```python
from build123d import *

# Parameters (mm, degrees)
SKETCH_1_R                   = 8.3
EXTRUDE_1_DEPTH              = 2.25
EXTRUDE_START                = 2
EXTRUDE_2_DEPTH              = 2
EXTRUDE_START_2              = 4.5
EXTRUDE_3_DEPTH              = 4.5
EXTRUDE_4_DEPTH              = 2
FILLET_1_R                   = 0.5
SKETCH_5_R                   = 1.85
EXTRUDE_5_DEPTH              = 0.5
HOLE_WIZARD_M2_1_D           = 2.1
HOLE_WIZARD_M2_1_CBORE_D     = 3.8
HOLE_WIZARD_M2_1_CBORE_DEPTH = 1
FILLET_2_R                   = 2


with BuildPart() as part:
    # ｽｹｯﾁ1 → ﾎﾞｽ - 押し出し1 (new body)
    with BuildSketch(Plane(origin=(0, 0, 0), x_dir=(1, 0, 0), z_dir=(0, 1, 0))):
        with BuildLine():
            ThreePointArc((13, 10.5), (0, 23.5), (-13, 10.5))
            Line((-13, 10.5), (-13, -13))
            Line((-13, -13), (13, -13))
            Line((13, -13), (13, 10.5))
        make_face()
        with Locations(Location((0, 10.5, 0), (0, 0, 270))):
            Circle(SKETCH_1_R, mode=Mode.SUBTRACT)
    extrude(amount=EXTRUDE_1_DEPTH)

    # ｽｹｯﾁ2 → ﾎﾞｽ - 押し出し2 (add)
    with BuildSketch(Plane.XZ.offset(EXTRUDE_START)):
        with BuildLine():
            Line((-12.649110641, -13.5), (-5.48292805, -13.5))
            ThreePointArc((-5.48292805, -13.5), (0, -16.75), (5.48292805, -13.5))
            Line((5.48292805, -13.5), (12.649110641, -13.5))
            ThreePointArc((12.649110641, -13.5), (0, -23.5), (-12.649110641, -13.5))
        make_face()
    extrude(amount=-EXTRUDE_2_DEPTH)

    # ｽｹｯﾁ3 → ﾎﾞｽ - 押し出し3 (add)
    with BuildSketch(Plane.XZ.offset(2).offset(EXTRUDE_START_2)):
        with BuildLine():
            Line((-9.38083152, -19.5), (-7.158910532, -19.5))
            ThreePointArc((-7.158910532, -19.5), (0, -22), (7.158910532, -19.5))
            Line((7.158910532, -19.5), (9.38083152, -19.5))
            ThreePointArc((9.38083152, -19.5), (0, -23.5), (-9.38083152, -19.5))
        make_face()
    extrude(amount=-EXTRUDE_3_DEPTH)

    # ｽｹｯﾁ4 → ﾎﾞｽ - 押し出し4 (add)
    with BuildSketch(Plane.XZ.offset(EXTRUDE_START)):
        with BuildLine():
            Line((-6.25, 6.25), (6.25, 6.25))
            Line((6.25, 6.25), (6.25, -10.5))
            ThreePointArc((6.25, -10.5), (0, -4.25), (-6.25, -10.5))
            Line((-6.25, -10.5), (-6.25, 6.25))
        make_face()
    extrude(amount=-EXTRUDE_4_DEPTH)

    # ﾌｨﾚｯﾄ1
    # the kernel refuses this fillet: 0.5 mm, written as the material it takes off along each edge
    with BuildSketch(Plane(origin=(5.48292805, -2.721925351, -13.5), x_dir=(1, 0, 0), z_dir=(0, 1, 0))) as fillet_1_piece_1:
        with BuildLine():
            CenterArc((0.28877014, 0.5), FILLET_1_R, 211.232929016, 58.767070984)
            ThreePointArc((-0.138763059, 0.240740741), (-0.068043475, 0.121141625), (0, 0))
            Line((0, 0), (0.28877014, 0))
        make_face()
    extrude(amount=3.443850702, mode=Mode.SUBTRACT)
    with BuildSketch(Plane(origin=(-5.48292805, -2.721925351, -13.5), x_dir=(-1, 0, 0), z_dir=(0, 1, 0))) as fillet_1_piece_2:
        with BuildLine():
            CenterArc((0.28877014, -0.5), FILLET_1_R, 90, 58.767070984)
            ThreePointArc((-0.138763059, -0.240740741), (-0.068043475, -0.121141625), (0, 0))
            Line((0, 0), (0.28877014, 0))
        make_face()
    extrude(amount=3.443850702, mode=Mode.SUBTRACT)
    with BuildSketch(Plane(origin=(-6.25, -10.838834765, -10.5), x_dir=(0, 0, 1), z_dir=(0, 1, 0))) as fillet_1_piece_3:
        with BuildLine():
            CenterArc((3.535533906, 0.5), FILLET_1_R, 121.586338097, 148.413661903)
            ThreePointArc((3.273642506, 0.925925926), (1.701034544, 0.235934696), (0, 0))
            Line((0, 0), (3.535533906, 0))
        make_face()
    extrude(amount=19.67766953, mode=Mode.SUBTRACT)
    with BuildSketch(Plane(origin=(6.25, -10.838834765, -10.5), x_dir=(0, 0, 1), z_dir=(0, 1, 0))) as fillet_1_piece_4:
        with BuildLine():
            CenterArc((3.535533906, -0.5), FILLET_1_R, 90, 148.413661903)
            ThreePointArc((3.273642506, -0.925925926), (1.701034544, -0.235934696), (0, 0))
            Line((0, 0), (3.535533906, 0))
        make_face()
    extrude(amount=19.67766953, mode=Mode.SUBTRACT)

    # ｽｹｯﾁ5 → ﾎﾞｽ - 押し出し5 (add)
    with BuildSketch(Plane.XZ):
        with Locations(Location((-10.5, 10.5, 0), (0, 0, 90))):
            Circle(SKETCH_5_R)
        with Locations(Location((10.5, 10.5, 0), (0, 0, 90))):
            Circle(SKETCH_5_R)
        with Locations(Location((-10.5, -10.5, 0), (0, 0, 90))):
            Circle(SKETCH_5_R)
        with Locations(Location((10.5, -10.5, 0), (0, 0, 90))):
            Circle(SKETCH_5_R)
    extrude(amount=EXTRUDE_5_DEPTH)

    # M2 丸平ねじ用座ぐり穴1 (through all)
    with Locations(Plane(origin=(0, 2.25, 0), x_dir=(1, 0, 0), z_dir=(0, 1, 0))):
        with Locations((10.5, 10.5), (-10.5, 10.5), (-10.5, -10.5), (10.5, -10.5)):
            CounterBoreHole(HOLE_WIZARD_M2_1_D / 2, HOLE_WIZARD_M2_1_CBORE_D / 2, HOLE_WIZARD_M2_1_CBORE_DEPTH)

    # ﾌｨﾚｯﾄ2
    fillet_2_edges = [part.edges().sort_by_distance(p)[0] for p in [
        (13, 1.125, 13),
        (-13, 1.125, 13),
    ]]
    fillet(fillet_2_edges, radius=FILLET_2_R)


solid = part.part
```
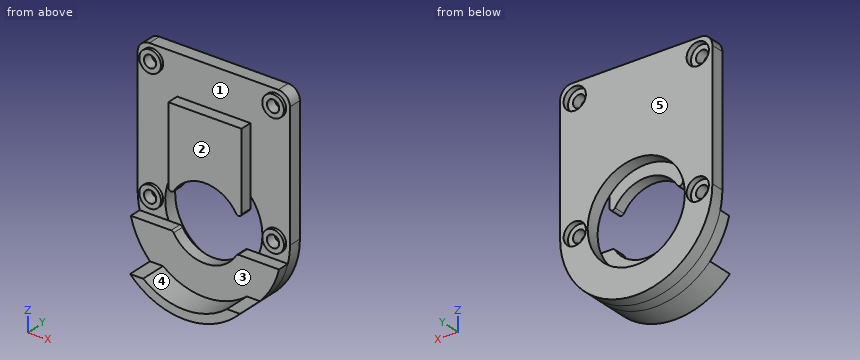
Source: CAD feature listing. Evaluate the final solid. Frame: model axes, mm. Face numbers are marked on the shaded views. A direction names the side the tool comes from. Coordinates: 2 decimals unless noted, no trailing zeros. Write each loop counter-clockwise with the first axis right and the second up, starting at its lowest first coordinate (ties: lowest second). Pieces come first, ordered by that corner, then holes. Notation, with made-up numbers: M 16.25,9.25 L 45.25,9.25 A26 ccw 45.25,36.25 Z; hole C -8.5,25.25 d6. An arc over 180 degrees is marked long. Answer as a JSON object with one key per item and string values.
1. Contact query for flat-ended pins moving along their axis: P1, Ø6, axis at x = 10.5, z = -10.5, coming from the +Y side; P2, Ø10, axis at x = 7.5, z = -11, coming from the -Y side; P3, Ø1.8, axis at x = 11.5, z = 10.5, coming from the -Y side; P4, Ø1.8, axis at x = 9, y = -4.5, coming from the +Z side. Output: stop coordinate, or through.
Evaluation:
{"P1": "y = 2.25", "P2": "y = -2", "P3": "y = -0.5", "P4": "z = -19.5"}
2. Cut plane C-C on x = 10.5. State how many separate pieces and enclosed holes the cut face has, plus the area to 3 significant figures.
Evaluation:
{"separate pieces": "3", "enclosed holes": "0", "area": "68.2 mm^2"}
3. Cut plane A-A on y = 1.75. Output: boundary loops of the cut face in (x, z).
Evaluation:
{"outline": "M -13,-10.5 A13 ccw 13,-10.5 L 13,11 A2 ccw 11,13 L -11,13 A2 ccw -13,11 Z; hole C -10.5,-10.5 d3.8; hole C -10.5,10.5 d3.8; hole C 0,-10.5 d16.6; hole C 10.5,-10.5 d3.8; hole C 10.5,10.5 d3.8"}
4. Access query for the marked faces 4 and 5. Directions: +Z, -Z, +X, -X, +Y, -Y. A direction counts if a zero-diameter tool reaches every point of the face in a straight line with its end or side. Return the directions, or none.
Evaluation:
{"face 4": "+Z, -Y", "face 5": "+Z, -Z, +X, -X, +Y"}
5. Ray query, L1, parallel to X at y = 0.5, z = -10.5; L2, parallel to Z at x = 0, y = 1.7; L3, parallel to Z at x = -10.5, y = 2. Return the intervals inside material, ascending.
Evaluation:
{"L1": "-13 to -11.55, -9.45 to -8.3, 8.3 to 9.45, 11.55 to 13", "L2": "-23.5 to -18.8, -2.2 to 13", "L3": "-18.16 to -12.4, -8.6 to 8.6, 12.4 to 13"}
6. Cut plane D-D on z = -14.5. Output: boundary loops of the cut face in (x, y).
Evaluation:
{"outline": "M -12.37,-2 L -4.8,-2 L -4.8,0 L -7.27,0 L -7.27,2.25 L -12.37,2.25 Z; M 4.8,-2 L 12.37,-2 L 12.37,2.25 L 7.27,2.25 L 7.27,0 L 4.8,0 Z"}
7. Draft query along X for the marked faces 1, 2 and 3. Return one class per face: released by +X, released by -X, zero draft, split by the parting line, or undercut.
Evaluation:
{"face 1": "undercut", "face 2": "zero draft", "face 3": "undercut"}
8. Cut plane B-B on x = 0. Output: boundary loops of the cut face in (y, z).
Evaluation:
{"outline": "M -6.5,-23.5 L 2.25,-23.5 L 2.25,-18.8 L 0,-18.8 L 0,-16.75 L -2,-16.75 L -2,-22 L -6.5,-22 Z; M -2,-4.25 L 0,-4.25 L 0,-2.2 L 2.25,-2.2 L 2.25,13 L 0,13 L 0,6.25 L -2,6.25 Z"}
